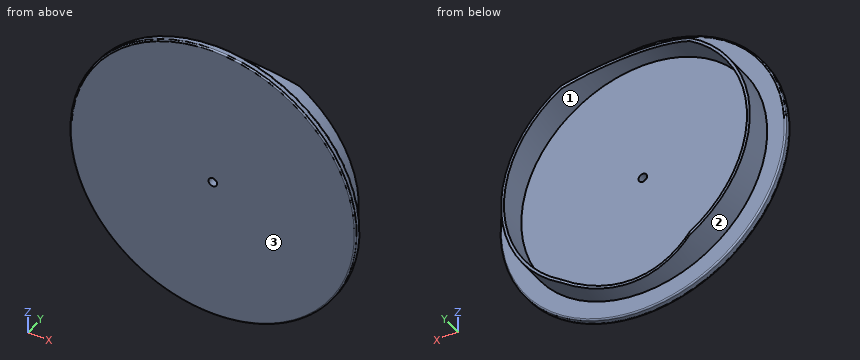
```python
from build123d import *

# Parameters (mm, degrees)
SKETCH2_R               = 100
SKETCH2_R_2             = 87
SKETCH2_R_3             = 85
BOSS_EXTRUDE1_DEPTH     = 5
SKETCH2_3_R             = 87
SKETCH2_3_R_2           = 85
BOSS_EXTRUDE2_DEPTH     = 25
CUT_EXTRUDE1_DEPTH      = 144.614066163
CUT_EXTRUDE1_DEPTH_BACK = 144.614066163
SKETCH4_R               = 3
CUT_EXTRUDE2_DEPTH      = 144.614066181
FILLET1_R               = 1


with BuildPart() as part:
    # Sketch2 → Boss-Extrude1 (new body)
    # profile 1 of 3: a face of its own
    with BuildSketch(Plane(origin=(0, 0, 0), x_dir=(1, 0, 0), z_dir=(0, 1, 0))):
        with Locations(Location((0, 0, 0), (0, 0, 270))):
            Circle(SKETCH2_R)
        Circle(SKETCH2_R_2, mode=Mode.SUBTRACT)
    # profile 2 of 3: a face of its own
    with BuildSketch(Plane(origin=(0, 0, 0), x_dir=(1, 0, 0), z_dir=(0, 1, 0))):
        Circle(SKETCH2_R_2)
        Circle(SKETCH2_R_3, mode=Mode.SUBTRACT)
    # profile 3 of 3: a face of its own
    with BuildSketch(Plane(origin=(0, 0, 0), x_dir=(1, 0, 0), z_dir=(0, 1, 0))):
        Circle(SKETCH2_R_3)
    extrude(amount=BOSS_EXTRUDE1_DEPTH)

    # Sketch2_3 → Boss-Extrude2 (add)
    with BuildSketch(Plane(origin=(0, 0, 0), x_dir=(1, 0, 0), z_dir=(0, 1, 0))):
        with Locations(Location((0, 0, 0), (0, 0, 270))):
            Circle(SKETCH2_3_R)
        with Locations(Location((0, 0, 0), (0, 0, 270))):
            Circle(SKETCH2_3_R_2, mode=Mode.SUBTRACT)
    extrude(amount=BOSS_EXTRUDE2_DEPTH)

    # Sketch3 → Cut-Extrude1 (cut, two sides: drawn at the far end of the back side and taken through both)
    with BuildSketch(Plane.XY.offset(-CUT_EXTRUDE1_DEPTH_BACK)):
        with BuildLine():
            Line((-45, 25), (-45, 27.803999392))
            Line((-45, 27.803999392), (45, 27.803999392))
            Line((45, 27.803999392), (45, 25))
            ThreePointArc((45, 25), (0, 16.983491439), (-45, 25))
        make_face()
    extrude(amount=CUT_EXTRUDE1_DEPTH + CUT_EXTRUDE1_DEPTH_BACK, mode=Mode.SUBTRACT)

    # Sketch4 → Cut-Extrude2 (cut, through all)
    with BuildSketch(Plane.XZ):
        with Locations(Location((0, 0, 0), (0, 0, 270))):
            Circle(SKETCH4_R)
    extrude(amount=-CUT_EXTRUDE2_DEPTH, mode=Mode.SUBTRACT)

    # Fillet1
    fillet1_edges = [part.edges().sort_by_distance(p)[0] for p in [
        (0, 0, -100),
        (0, 5, -100),
    ]]
    fillet(fillet1_edges, radius=FILLET1_R)


solid = part.part
```
Design review of the part built by this model. Coordinates are the model's own, in mm. Face numbers are marked on the shaded views. Coordinates: 2 decimals unless noted, no trailing zeros. Order: outer loops, then holes, each group sorted by start corner. A loop starts at its lowest first (then second) coordinate and runs counter-clockwise, first axis right, second up.
1) Take a section at A-A, the plane x = 0. Give the boundary of the cut face in (y, z).
2) Wall thickness on line 1 along X through (y, z) = (1.8, 0); line 2 along X through (y, z) = (11.25, 0); line 3 along Y through (x, z) = (-12.5, -46): over which ranges is each line inside the solid? List them lowest first.
3) Take a section at B-B, the plane z = 0. Give the boundary of the cut face in (x, y), and give its area (3 significant figures).
4) Clearance check with flat-ended pins moving along their axes: pin 1 (1.5 mm diameter, centred on x = 37, y = 11, fed in from -Z); pin 2 (6 mm diameter, centred on y = 19.5, z = -9.5, fed in from +X); pin 3 (1.5 mm diameter, centred on x = -20, z = -22, fed in from +Y); pin 4 (5.5 mm diameter, centred on x = 0, z = 0, fed in from -Y). State where each tip first meets the part, or that it passes through.
5) Take a section at C-C, the plane y = 10.5. Give the boundary of the cut face in (x, z).
6) Mouldability with a two-part tool opening along Z and no side actions: class the marked faces 1, 2 and 3 as +Z half, -Z half, draft (parallel to the pull), parting line (faces both ways), or undercut.
Returned:
1. outline: (0, -99) arc R1 ccw to (1, -100) - (4, -100) arc R1 ccw to (5, -99) - (5, -87) - (16.98, -87) - (16.98, -85) - (5, -85) - (5, -3) - (0, -3) - close; (0, 3) - (5, 3) - (5, 85) - (16.98, 85) - (16.98, 87) - (5, 87) - (5, 99) arc R1 ccw to (4, 100) - (1, 100) arc R1 ccw to (0, 99) - close
2. line 1: x = -100 to -3, 3 to 100
2. line 2: x = -87 to -85, 85 to 87
2. line 3: y = 0 to 5
3. outline: (-100, 1) arc R1 ccw to (-99, 0) - (-3, 0) - (-3, 5) - (-85, 5) - (-85, 25) - (-87, 25) - (-87, 5) - (-99, 5) arc R1 ccw to (-100, 4) - close; (3, 0) - (99, 0) arc R1 ccw to (100, 1) - (100, 4) arc R1 ccw to (99, 5) - (87, 5) - (87, 25) - (85, 25) - (85, 5) - (3, 5) - close
3. area: 1,050 mm2
4. pin 1: stops at z = -79.09
4. pin 2: stops at x = 86.76
4. pin 3: stops at y = 5
4. pin 4: passes through
5. outline: circle Ø174 at (0, 0); hole circle Ø170 at (0, 0)
6. face 1: undercut
6. face 2: parting line
6. face 3: draft
